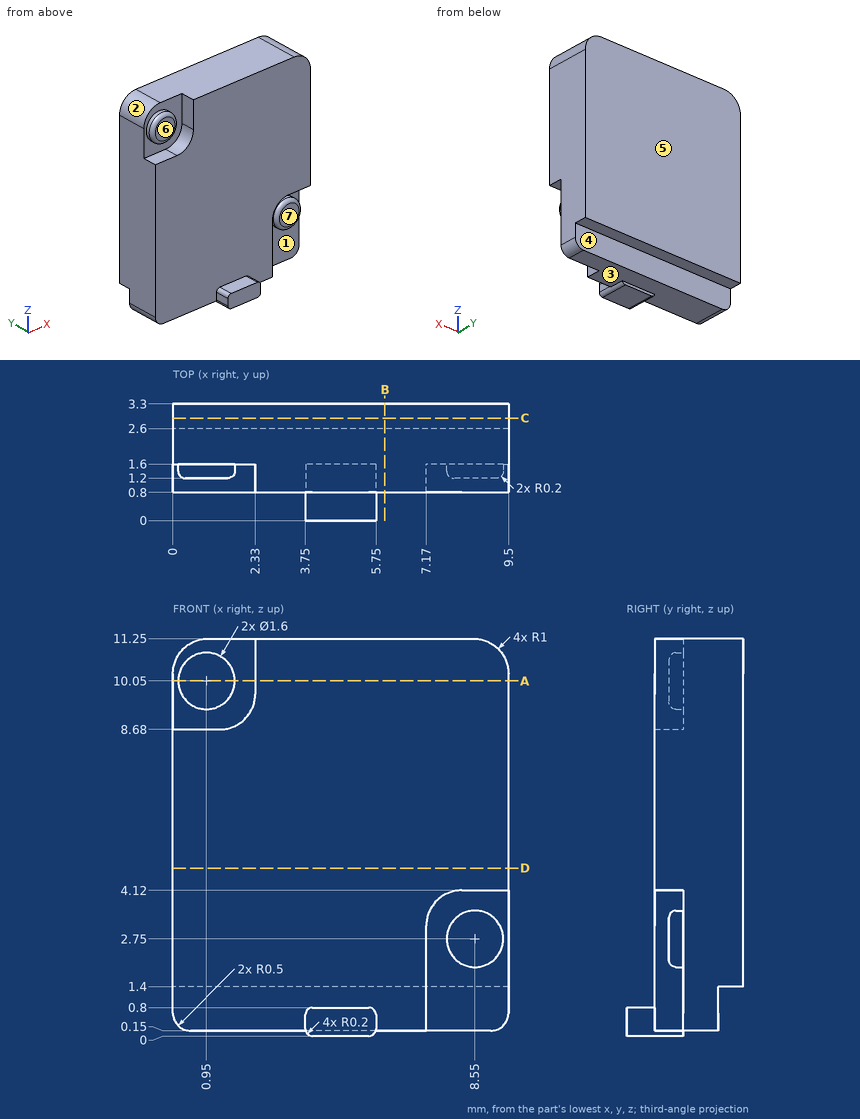
Geometry check sheet. Reference: drawing and pictorial views, mm from the part's lowest x, y, z. A direction names the side the tool comes from. Give positions to 0.01 mm unless a question says otherwise; leave off trailing zeros. Order: outer loops, then holes, each group sorted by start corner. A loop starts at its lowest first (then second) coordinate and runs counter-clockwise, first axis right, second up. Notation, with made-up numbers: M 85,28.5 L 127,28.5 A19 ccw 127,45.5 Z; hole C 34,17.25 d5. An arc over 180 degrees is marked long. Answer as CSV lines item,"result". Start each with the question number.
Item 1: Cross-section at D-D on z = 4.75. Enter the section's corners in (x, y).
Item 2: Gauge pin test, flat ends, axial feed: P1, Ø0.9, axis at x = 1, y = 1, coming from the +Z side; P2, Ø0.7, axis at x = 8, z = 2, coming from the -Y side; P3, Ø1, axis at x = 5.5, z = 0.5, coming from the +Y side. Record the tip position at first contact, or that the pin passes through.
Item 3: Thickness scan on line 1 (Y direction, x = 3, z = 8.5); line 2 (Z direction, x = 4.25, y = 1.7); line 3 (Y direction, x = 8, z = 4). Record the ranges inside material, lowest first. Write a range as [from, to].
Item 4: Mould release check, pull along Z, two halves, no side actions. Record for the marked faces 1, 2, 3 and 4: +Z half, -Z half, draft (parallel to the pull), parting line (faces both ways), or undercut.
Item 5: Cross-section at A-A on z = 10.05. Enter the section's corners in (x, y), plus the area to 3 significant figures.
Item 6: Cross-section at C-C on y = 2.9. Enter the section's corners in (x, z).
Item 7: Cross-section at B-B on x = 6. Enter the section's corners in (y, z).
Item 8: Tool access check on the marked faces 5, 6 and 7. Record the directions out of +Z, -Z, +X, -X, +Y, -Y that give a thin tool (end or side, any length) a straight path to the whole face; none if there is none.
Established:
1,outline,"M 0,0.8 L 9.5,0.8 L 9.5,3.3 L 0,3.3 Z"
2,P1,"stops at z = 10.85"
2,P2,"stops at y = 1.2"
2,P3,"stops at y = 2.6"
3,line 1,"y = [0.8, 3.3]"
3,line 2,"z = [0.15, 11.25]"
3,line 3,"y = [1.6, 3.3]"
4,face 1,"undercut"
4,face 2,"+Z half"
4,face 3,"-Z half"
4,face 4,"draft"
5,outline,"M 0,1.6 L 0.15,1.6 L 0.15,1.4 A0.2 ccw 0.35,1.2 L 1.55,1.2 A0.2 ccw 1.75,1.4 L 1.75,1.6 L 2.33,1.6 L 2.33,0.8 L 9.5,0.8 L 9.5,3.3 L 0,3.3 Z"
5,area,"22.5 mm^2"
6,outline,"M 0,1.4 L 9.5,1.4 L 9.5,10.25 A1 ccw 8.5,11.25 L 1,11.25 A1 ccw 0,10.25 Z"
7,outline,"M 0.8,0.15 L 2.6,0.15 L 2.6,1.4 L 3.3,1.4 L 3.3,11.25 L 0.8,11.25 Z"
8,face 5,"+Z, -Z, +X, -X, +Y"
8,face 6,"+Z, -X, -Y"
8,face 7,"-Z, +X, -Y"
